```python
from build123d import *

# Parameters (mm, degrees)
F0_R         = 12.7
F0_R_2       = 3.429
F1_DEPTH     = 5.08
F2_SIZE      = 3.175
F3_DEPTH     = 1.27
F4_R         = 9.525
F4_R_2       = 7.747
F5_DEPTH     = 20.32
F6_R         = 7.747
F7_DEPTH     = 25.4
F8_T4_DEPTH  = 81.8307478943
F8_S5_R      = 9.525
F8_T6_DEPTH  = 43
F9_W         = 6.35
F9_H         = 11.43
F10_DEPTH    = 14.224
F11_T1_DEPTH = 6.35
F12_R        = 3.302
F13_DEPTH    = 12.7
F14_SIZE     = 0.635


# Not quite as in the source:
# - a fillet or chamfer that OpenCascade refuses, or shapes differently, is made with other operations: its cross-section is extruded or revolved along the edge and cut away or added


with BuildPart() as f1:
    # F0 (on Top) → F1 (new body)
    with BuildSketch(Plane.XY):
        Circle(F0_R)
        Circle(F0_R_2, mode=Mode.SUBTRACT)
    extrude(amount=F1_DEPTH)

    # F2
    f2_edges = [f1.edges().sort_by_distance(p)[0] for p in [
        (-12.7, 0, 5.08),
    ]]
    chamfer(f2_edges, length=F2_SIZE)

    # F3 (add): a face of the model
    f3_faces = [f1.faces().sort_by_distance(p)[0] for p in [
        (-9.2555923164, 0, 5.08),
    ]]
    extrude(f3_faces, amount=F3_DEPTH)

    # F4 (on face) → F5 (join)
    with BuildSketch(Plane.XY.offset(6.35)):
        Circle(F4_R)
        Circle(F4_R_2, mode=Mode.SUBTRACT)
    extrude(amount=F5_DEPTH)

    # F6 (on face) → F7 (join)
    with BuildSketch(Plane.XY.offset(26.67)):
        with BuildLine():
            ThreePointArc((9.525, 0), (4.7677946163, 8.2458328565), (-4.7519048812, 8.255))
            ThreePointArc((-4.7519048812, 8.255), (-9.525, 0), (-4.7519048812, -8.255))
            ThreePointArc((-4.7519048812, -8.255), (4.7677946163, -8.2458328565), (9.525, 0))
        make_face()
        Circle(F6_R, mode=Mode.SUBTRACT)
        with BuildLine():
            ThreePointArc((-4.7519048812, -8.255), (-9.525, 0), (-4.7519048812, 8.255))
            Line((-4.7519048812, 8.255), (-17.6784, 8.255))
            Line((-17.6784, 8.255), (-17.6784, -8.255))
            Line((-17.6784, -8.255), (-4.7519048812, -8.255))
        make_face()
    extrude(amount=F7_DEPTH)

    # F8: chamfer of 12.7 on 1 edges, made by hand


with BuildPart() as f8_tool2:
    # F8_s3 → F8_t4 (new body)
    with BuildSketch(Plane.XZ.offset(-40.9153739472)):
        Polygon((-4.9784, 26.67), (-17.6784, 39.37), (-17.6784, 26.67), align=None)
    extrude(amount=F8_T4_DEPTH)

    # F8_s5 → F8_t6 (cut, symmetric)
    with BuildSketch(Plane.XY.offset(33)):
        Circle(F8_S5_R)
    extrude(amount=F8_T6_DEPTH, both=True, mode=Mode.SUBTRACT)


with BuildPart() as f1_1:
    add(f1.part)

    # F8_t1: cut F8_tool2
    add(f8_tool2.part, mode=Mode.SUBTRACT)

    # F9 (on face) → F10 (cut)
    with BuildSketch(Plane.XY.offset(52.07)):
        with Locations((-12.4714, 0)):
            Rectangle(F9_W, F9_H)
    extrude(amount=-F10_DEPTH, mode=Mode.SUBTRACT)

    # F11: chamfer of 3.302 x 5.7192317666 on 2 edges, made by hand

    # F11_s2 → F11_t1 (join)
    with BuildSketch(Plane.YZ.offset(-15.6464)):
        Polygon((5.715, 41.148), (-0.0042317666, 37.846), (5.715, 37.846), align=None)
        Polygon((-5.715, 41.148), (0.0042317666, 37.846), (-5.715, 37.846), align=None)
    extrude(amount=F11_T1_DEPTH)

    # F12 (on face) → F13 (cut, symmetric)
    with BuildSketch(Plane.YZ.offset(-15.6464)):
        with Locations((0, 44.4475567884)):
            Circle(F12_R)
    extrude(amount=F13_DEPTH, both=True, mode=Mode.SUBTRACT)

    # F14
    f14_edges = [f1_1.edges().sort_by_distance(p)[0] for p in [
        (-7.747, 0, 52.07),
    ]]
    chamfer(f14_edges, length=F14_SIZE)


solid = f1_1.part
```
Design review of the part built by this model. Coordinates are the model's own, in mm. A direction names the side the tool comes from. Give positions to 0.01 mm unless a question says otherwise; leave off trailing zeros. Write each loop counter-clockwise with the first axis right and the second up, starting at its lowest first coordinate (ties: lowest second). Pieces come first, ordered by that corner, then holes. Notation, with made-up numbers: (19.5, -6) - (52.5, -6) arc R18 ccw to (52.5, 29) - close; hole circle Ø10 at (49, -7). An arc over 180 degrees is marked (long way). Return JSON: item names as keys, results as strings. Group by question number.
(1) We need section C-C, the plane z = 7. Give the boundary of the cut face in (x, y) (3 decimals), then the cut area to 3 significant figures.
(2) We need section B-B, the plane z = 32.5. Give the boundary of the cut face in (x, y) (3 decimals), then the cut area to 3 significant figures.
(3) Mouldability with a two-part tool opening along X and no side actions: class faces 1 (the flat face through (-13, 5.715, 47)), 2 (the flat face through (3, -2, 6.35)), 3 (the cylindrical face through (-16.65, 1.78, 47.23)), 4 (the flat face through (-17.678, 0, 48)) as +X half, -X half, draft (parallel to the pull), parting line (faces both ways), or undercut.
(4) We need section A-A, the plane x = 0. Give the boundary of the cut face in (y, z) (3 decimals), then the cut area to 3 significant figures.
(5) To check wall thickness, follow probe 1 along X at (y, z) = (0, 31) (3 decimals); probe 2 along Z at (x, y) = (-16.15, 0). State the ranges of each line that lie inside material, in increasing order.
(6) Machinability: for faces 5 (the cylindrical face through (-8.39, -2.434, 46.679)), 6 (the flat face through (-9.296, 0, 48)), 7 (the flat face through (-11, -8.255, 42)), 8 (the cylindrical face through (-2.75, -12.4, 0.94)), which of the approach directions +Z, -Z, +X, -X, +Y, -Y give a long, thin tool a straight path to every point of the face, cutting with its end or side? Answer none if there is none.
(7) Insertion check: pin 1 (7 mm diameter, centred on x = -14, z = 47, fed in from -Y) (3 decimals); pin 2 (4 mm diameter, centred on y = 0, z = 45.5, fed in from +X) (3 decimals); pin 3 (5 mm diameter, centred on y = 4.5, z = 31, fed in from +X); pin 4 (4 mm diameter, centred on x = 0, y = 0, fed in from -Z). Each pin has a flat end and moves straight along its axis. Give the tip position at first contact, or say it passes through.
Reported:
{
 "1": {"outline": "circle Ø19.05 at (0, 0); hole circle Ø15.494 at (0, 0)", "area": "96.5 mm2"},
 "2": {"outline": "(-10.808, -8.255) - (-4.752, -8.255) arc R9.525 ccw (long way) to (-4.752, 8.255) - (-10.808, 8.255) - close; hole circle Ø15.494 at (0, 0)", "area": "141 mm2"},
 "3": {"face 1": "undercut", "face 2": "undercut", "face 3": "draft", "face 4": "-X half"},
 "4": {"outline": "(-12.7, 0) - (-3.429, 0) - (-3.429, 6.35) - (-7.747, 6.35) - (-7.747, 51.435) - (-8.382, 52.07) - (-9.525, 52.07) - (-9.525, 5.08) - (-12.7, 1.905) - close; (3.429, 0) - (12.7, 0) - (12.7, 1.905) - (9.525, 5.08) - (9.525, 52.07) - (8.382, 52.07) - (7.747, 51.435) - (7.747, 6.35) - (3.429, 6.35) - close", "area": "262 mm2"},
 "5": {"probe 1": "x = -9.525 to -7.747, 7.747 to 9.525", "probe 2": "z = 37.84 to 41.15, 47.75 to 52.07"},
 "6": {"face 5": "-X", "face 6": "+Z", "face 7": "+Z, -X, -Y", "face 8": "-Z"},
 "7": {"pin 1": "stops at y = -8.255", "pin 2": "stops at x = 9.525", "pin 3": "stops at x = 9.31", "pin 4": "passes through"}
}
